from build123d import *

# Parameters (mm, degrees)
BOSS_EXTRUDE2_DEPTH = 63.5
SKETCH4_R           = 1.27
CUT_EXTRUDE1_DEPTH  = 2.54
CUT_EXTRUDE2_START  = -2.54
SKETCH5_R           = 1.27
CUT_EXTRUDE2_DEPTH  = 2.54


with BuildPart() as part:
    # Sketch3 → Boss-Extrude2 (new, symmetric)
    with BuildSketch(Plane.XY):
        Polygon((-63.5, 12.7), (-63.5, -12.7), (63.5, -12.7), (63.5, 12.7), (58.7375, 12.7), (58.7375, -7.9375), (-58.7375, -7.9375), (-58.7375, 12.7), align=None)
    extrude(amount=BOSS_EXTRUDE2_DEPTH, both=True)

    # Sketch4 → Cut-Extrude1 (cut)
    with BuildSketch(Plane.XY.offset(63.5)):
        with Locations((-60.452, 7.62)):
            Circle(SKETCH4_R)
        with Locations(Location((59.563, -9.652, 0), (0, 0, 180))):
            Circle(SKETCH4_R)
        with Locations((60.452, 7.62)):
            Circle(SKETCH4_R)
        with Locations((-21.463, -9.652)):
            Circle(SKETCH4_R)
        with Locations((21.463, -9.652)):
            Circle(SKETCH4_R)
        with Locations((-59.563, -9.652)):
            Circle(SKETCH4_R)
    extrude(amount=-CUT_EXTRUDE1_DEPTH, mode=Mode.SUBTRACT)

    # Sketch5 → Cut-Extrude2 (cut)
    with BuildSketch(Plane(origin=(0, 0, -63.5), x_dir=(-1, 0, 0), z_dir=(0, 0, -1)).offset(CUT_EXTRUDE2_START)):
        with Locations((-59.563, -9.652)):
            Circle(SKETCH5_R)
        with Locations(Location((-60.452, 7.62, 0), (0, 0, 180))):
            Circle(SKETCH5_R)
        with Locations(Location((-21.463, -9.652, 0), (0, 0, 180))):
            Circle(SKETCH5_R)
        with Locations(Location((21.463, -9.652, 0), (0, 0, 180))):
            Circle(SKETCH5_R)
        with Locations(Location((60.452, 7.62, 0), (0, 0, 180))):
            Circle(SKETCH5_R)
        with Locations(Location((59.563, -9.652, 0), (0, 0, 180))):
            Circle(SKETCH5_R)
    extrude(amount=CUT_EXTRUDE2_DEPTH, mode=Mode.SUBTRACT)


solid = part.part
Check sheet for the modelled part. Datum: model origin and axes. Units: mm. A direction names the side the tool comes from. Round coordinates to 2 decimals unless told otherwise and drop trailing zeros. Order: outer loops, then holes, each group sorted by start corner. A loop starts at its lowest first (then second) coordinate and runs counter-clockwise, first axis right, second up.
Q1. Draft check along X on faces 3 (the face through (58.738, 3, 1)), 4 (the face through (-63.5, 0, 1)), 5 (the face through (-61, 12.7, 1)). Enter one of: pulls with the +X half, pulls with the -X half, needs draft (parallel to the pull), parting line crosses it, or undercut.
Filled sheet:
face 3: undercut
face 4: pulls with the -X half
face 5: needs draft
Q2. Cross-section at A-A, the plane y = 2.25. Enter the section's corners in (x, z), plus the area to 3 significant figures.
Filled sheet:
outline: (-63.5, -63.5) - (-58.74, -63.5) - (-58.74, 63.5) - (-63.5, 63.5) - close; (58.74, -63.5) - (63.5, -63.5) - (63.5, 63.5) - (58.74, 63.5) - close
area: 1,210 mm2
Q3. Cross-section at C-C, the plane x = -46. Enter the section's corners in (y, z), plus the area to 3 significant figures.
Filled sheet:
outline: (-12.7, -63.5) - (-7.94, -63.5) - (-7.94, 63.5) - (-12.7, 63.5) - close
area: 605 mm2
Q4. Cross-section at B-B, the plane z = 21. Enter the section's corners in (x, y).
Filled sheet:
outline: (-63.5, -12.7) - (63.5, -12.7) - (63.5, 12.7) - (58.74, 12.7) - (58.74, -7.94) - (-58.74, -7.94) - (-58.74, 12.7) - (-63.5, 12.7) - close
Q5. Set-up check for faces 1 (the face through (0, -9, 63.5)), 2 (the face through (1, -7.938, 1)): record each of +Z, -Z, +X, -X, +Y, -Y from which the full face is reachable in a straight line by a thin tool's end or side.
Filled sheet:
face 1: +Z, +X, -X, +Y, -Y
face 2: +Z, -Z, +Y
Q6. Scan lines: L1, parallel to X at y = 3.5, z = 26; L2, parallel to Y at x = -23.5, z = 12. Record each from-to range of solid material in increasing order.
Filled sheet:
L1: x = -63.5 to -58.74, 58.74 to 63.5
L2: y = -12.7 to -7.94
Q7. Depth check by flat-ended pin: P1, Ø1.3, axis at x = 21.5, y = -10, coming from the +Z side; P2, Ø2, axis at x = 21.463, y = -9.652, coming from the -Z side; P3, Ø3, axis at x = 21.463, y = -9.652, coming from the +Z side; P4, Ø1, axis at x = -15, z = -9.5, coming from the +Y side. Enter the tip coordinate at first touch or a pass-through.
Filled sheet:
P1: stops at z = 60.96
P2: stops at z = -60.96
P3: stops at z = 63.5
P4: stops at y = -7.94
